Work out the finished part from the listing and answer in its coordinate system (mm). A direction names the side the tool comes from. Give positions to 0.01 mm unless a question says otherwise; leave off trailing zeros. Write each loop counter-clockwise with the first axis right and the second up, starting at its lowest first coordinate (ties: lowest second). Pieces come first, ordered by that corner, then holes. Notation, with made-up numbers: (-21.75, 40) - (15.25, 40) arc R20 ccw to (15.25, 63) - close; hole circle Ø6 at (72, -34). An arc over 180 degrees is marked (long way). Write item = value, one per line.
from build123d import *

# Parameters (mm, degrees)
BOSS_EXTRUDE1_DEPTH      = 110
SKETCH2_R                = 4
SKETCH2_R_2              = 2.75
CUT_EXTRUDE1_DEPTH       = 9
CUT_EXTRUDE2_DEPTH       = 6
BOSS_EXTRUDE2_DEPTH      = 3
BOSS_EXTRUDE2_DEPTH_BACK = 2
BOSS_EXTRUDE4_DEPTH      = 2
BOSS_EXTRUDE4_DEPTH_BACK = 3
FILLET1_R                = 2


with BuildPart() as part:
    # Sketch1 → Boss-Extrude1 (new body)
    with BuildSketch(Plane.XY):
        Polygon((0, 0), (60, 0), (60, 6), (9, 6), (9, 70), (0, 70), align=None)
    extrude(amount=BOSS_EXTRUDE1_DEPTH)

    # Sketch2 → Cut-Extrude1 (cut)
    with BuildSketch(Plane.ZY):
        with Locations((55, 36)):
            Circle(SKETCH2_R)
        with Locations((78.57, 59.57)):
            Circle(SKETCH2_R_2)
        with Locations((31.43, 59.57)):
            Circle(SKETCH2_R_2)
        with Locations((31.43, 12.43)):
            Circle(SKETCH2_R_2)
        with Locations((78.57, 12.43)):
            Circle(SKETCH2_R_2)
    extrude(amount=-CUT_EXTRUDE1_DEPTH, mode=Mode.SUBTRACT)

    # Sketch3 → Cut-Extrude2 (cut)
    with BuildSketch(Plane(origin=(0, 6, 0), x_dir=(1, 0, 0), z_dir=(0, 1, 0))):
        with BuildLine():
            Line((25, -14.2), (50, -14.2))
            ThreePointArc((50, -14.2), (53.3, -17.5), (50, -20.8))
            Line((50, -20.8), (25, -20.8))
            ThreePointArc((25, -20.8), (21.7, -17.5), (25, -14.2))
        make_face()
        with BuildLine():
            Line((25, -39.2), (50, -39.2))
            ThreePointArc((50, -39.2), (53.3, -42.5), (50, -45.8))
            Line((50, -45.8), (25, -45.8))
            ThreePointArc((25, -45.8), (21.7, -42.5), (25, -39.2))
        make_face()
        with BuildLine():
            Line((25, -64.2), (50, -64.2))
            ThreePointArc((50, -64.2), (53.3, -67.5), (50, -70.8))
            Line((50, -70.8), (25, -70.8))
            ThreePointArc((25, -70.8), (21.7, -67.5), (25, -64.2))
        make_face()
        with BuildLine():
            Line((25, -89.2), (50, -89.2))
            ThreePointArc((50, -89.2), (53.3, -92.5), (50, -95.8))
            Line((50, -95.8), (25, -95.8))
            ThreePointArc((25, -95.8), (21.7, -92.5), (25, -89.2))
        make_face()
    extrude(amount=-CUT_EXTRUDE2_DEPTH, mode=Mode.SUBTRACT)

    # Sketch7 → Boss-Extrude2 (add, two sides: drawn at the far end of the back side and taken through both)
    with BuildSketch(Plane.XY.offset(102).offset(-BOSS_EXTRUDE2_DEPTH_BACK)):
        Polygon((9, 56), (34, 6), (9, 6), align=None)
    extrude(amount=BOSS_EXTRUDE2_DEPTH + BOSS_EXTRUDE2_DEPTH_BACK)

    # Sketch9 → Boss-Extrude4 (add, two sides: drawn at the far end of the back side and taken through both)
    with BuildSketch(Plane.XY.offset(8).offset(-BOSS_EXTRUDE4_DEPTH_BACK)):
        Polygon((9, 56), (9, 6), (34, 6), align=None)
    extrude(amount=BOSS_EXTRUDE4_DEPTH + BOSS_EXTRUDE4_DEPTH_BACK)

    # Fillet1
    fillet1_edges = [part.edges().sort_by_distance(p)[0] for p in [
        (21.5, 31, 100),
        (21.5, 31, 105),
        (21.5, 31, 5),
        (21.5, 31, 10),
        (60, 3, 110),
        (4.5, 70, 110),
        (4.5, 70, 0),
        (60, 3, 0),
    ]]
    fillet(fillet1_edges, radius=FILLET1_R)


solid = part.part
1. For a pull along Z with two mould halves and no side action, classify faces 6 (the flat face through (7, 27, 0)), 7 (the cylindrical face through (4.437, 15.157, 78.212)), 8 (the flat face through (21.7, 30.6, 7.5)) as pulls with the +Z half, pulls with the -Z half, needs draft (parallel to the pull), parting line crosses it, or undercut.
Solution:
face_6 = pulls with the -Z half
face_7 = undercut
face_8 = needs draft
2. A tool of negligible diameter and unlimited length cuts with its end or side. For faces 1 (the flat face through (5, 70, 54)), 2 (the flat face through (15, 19, 105)), 3 (the flat face through (38, 3, 95.8)), 4 (the cylindrical face through (20.815, 31.095, 9.399)), 5 (the flat face through (15, 19, 5)), from which of +Z, -Z, +X, -X, +Y, -Y can it reach the whole face along a straight path? Write none if from no direction.
Solution:
face_1 = +Z, -Z, +X, -X, +Y
face_2 = +Z, +X, +Y
face_3 = +Y, -Y
face_4 = +X, +Y
face_5 = -Z, +X, +Y
3. Given pin 1 (7 mm diameter, centred on x = 23.5, y = 24.5, fed in from -Z); pin 2 (3.5 mm diameter, centred on y = 59.57, z = 31.43, fed in from +X); pin 3 (12 mm diameter, centred on x = 32, z = 40, fed in from -Y); pin 4 (5 mm diameter, centred on y = 22.5, z = 78, fed in from +X), each flat-ended and moving along its own axis, determine where each tip first touches the part or whether it passes through.
Solution:
pin_1 = 5
pin_2 = through
pin_3 = 0
pin_4 = 9
4. Straight lines are drawn through the part: line 1 (Y direction, x = 5.5, z = 78.57); line 2 (Z direction, x = 21, y = 20); line 3 (Y direction, x = 2, z = 55). For each, find the intervals that lie inside material, in ascending order.
Solution:
line_1 = 0 to 9.68, 15.18 to 56.82, 62.32 to 70
line_2 = 5 to 10, 100 to 105
line_3 = 0 to 32, 40 to 70
5. Find section A-A, the plane y = 59.57. Give the vertices of the cut face in (x, z), then the cut area to 3 significant figures.
Solution:
outline = (0, 0) - (9, 0) - (9, 28.68) - (0, 28.68) - close; (0, 34.18) - (9, 34.18) - (9, 75.82) - (0, 75.82) - close; (0, 81.32) - (9, 81.32) - (9, 110) - (0, 110) - close
area = 891 mm^2
6. Find section D-D, the plane z = 48. Give the vertices of the cut face in (x, y), then the cut area to 3 significant figures.
Solution:
outline = (0, 0) - (60, 0) - (60, 6) - (9, 6) - (9, 70) - (0, 70) - close
area = 936 mm^2
7. Find section C-C, the plane x = 38. Give the vertices of the cut face in (y, z).
Solution:
outline = (0, 0) - (6, 0) - (6, 14.2) - (0, 14.2) - close; (0, 20.8) - (6, 20.8) - (6, 39.2) - (0, 39.2) - close; (0, 45.8) - (6, 45.8) - (6, 64.2) - (0, 64.2) - close; (0, 70.8) - (6, 70.8) - (6, 89.2) - (0, 89.2) - close; (0, 95.8) - (6, 95.8) - (6, 110) - (0, 110) - close
8. Find section B-B, the plane z = 67.5. Give the vertices of the cut face in (x, y).
Solution:
outline = (0, 0) - (21.7, 0) - (21.7, 6) - (9, 6) - (9, 70) - (0, 70) - close; (53.3, 0) - (60, 0) - (60, 6) - (53.3, 6) - close
